Could you check a few things on this model? Use its own coordinates, in mm. Coordinates: 2 decimals unless noted, no trailing zeros. Write each loop counter-clockwise with the first axis right and the second up, starting at its lowest first coordinate (ties: lowest second). Pieces come first, ordered by that corner, then holes. Notation, with made-up numbers: (50.5, -29) - (55.5, -29) arc R27 ccw to (55.5, -4) - close; hole circle Ø11 at (-16.75, 0.5). An arc over 180 degrees is marked (long way). Answer as a JSON object with one key per item and string values. Group by question number.
1) If we section it at A-A (x = 37.1): Write out the boundary of the cut face in (y, z) (3 decimals).
2) Please list where this line runs through material, in increasing order: line 1 along Y through (x, z) = (37.65, 56) (3 decimals).
3) If we section it at B-B (z = 8): Write out the boundary of the cut face in (x, y) (3 decimals), plus the area to 3 significant figures.
4) Will this pin go through, and if not, where does the flat tip stop? pin 1 Ø1 at (x, z) = (37, 57.5) entering from -Y (3 decimals).
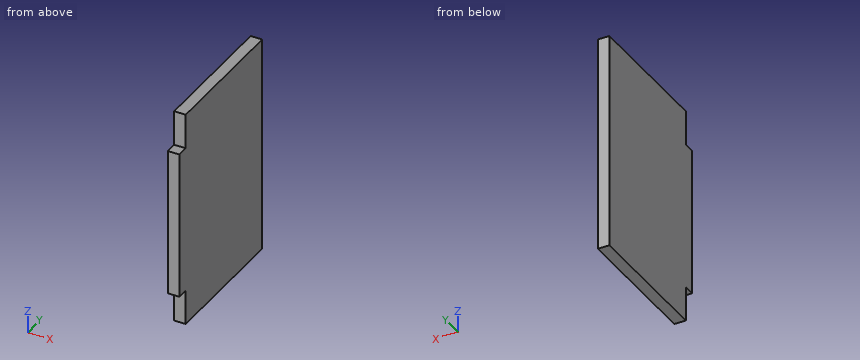
Autodesk Inventor part; units mm, degrees
ref_plane "YZ Plane" through (0, 0, 0) normal (1, 0, 0) x (0, 1, 0)
ref_plane "XZ Plane" through (0, 0, 0) normal (0, 1, 0) x (-1, 0, 0)
ref_plane "XY Plane" through (0, 0, 0) normal (0, 0, 1) x (1, 0, 0)
sketch "Sketch1" plane through (0, 0, 0) normal (0, 0, 1) x (1, 0, 0)
  line L0 (0, 0) -> (-3.175, 0)
  line L1 (-3.175, 0) -> (-3.175, 40.64)
  line L2 (-3.175, 40.64) -> (0, 40.64)
  line L3 (0, 40.64) -> (0, 0)
  line L4 (-41.275, -9.5758) -> (-3.175, -9.5758)
  line L5 (-3.175, -9.5758) -> (-3.175, 50.2158)
  line L6 (-3.175, 50.2158) -> (-41.275, 50.2158)
  line L7 (-41.275, 50.2158) -> (-41.275, -9.5758)
  point P0 (-22.225, 50.2158)
  point P1 (-22.225, -9.5758)
  point P2 (-3.175, 0)
  point P3 (-3.175, 40.64)
  dimension "d0" = 3.175
  dimension "d1" = 40.64
  dimension "d2" = 59.7916
  dimension "d3" = 9.5758
  dimension "d5" = 38.1
  dimension "d6" = 0
extrude "Extrusion1" add sketch "Sketch1" along normal blind 3.175
move or copy body "Move Body1" bodies to move or copy 1 copy no rotation origin (0, 0, 0) rotation axis (0, 0, 1) rotation angle -90 translate (-40.64, 40.64, 0)
move or copy body "Move Body2" bodies to move or copy 1 copy no rotation origin (0, 0, 0) rotation axis (0, -1, 0) rotation angle -90 translate (9.5758, 0, 9.5758)
move or copy body "Move Body3" bodies to move or copy 1 copy no translate (25.4, 0, 0)
properties part number "servo long side"
Here are the results:
{
 "1": {"outline": "(40.64, 9.576) - (43.815, 9.576) - (43.815, 0) - (81.915, 0) - (81.915, 59.792) - (43.815, 59.792) - (43.815, 50.216) - (40.64, 50.216) - close"},
 "2": {"line 1": "y = 43.815 to 81.915"},
 "3": {"outline": "(34.976, 43.815) - (38.151, 43.815) - (38.151, 81.915) - (34.976, 81.915) - close", "area": "121 mm²"},
 "4": {"pin 1": "stops at y = 43.815"}
}
